```python
from build123d import *

# Parameters (mm, degrees)
SKETCH1_W           = 120
SKETCH1_H           = 110
SKETCH1_W_2         = 98
SKETCH1_H_2         = 40.5
BOSS_EXTRUDE1_DEPTH = 5
SKETCH2_R           = 1.25
CUT_EXTRUDE1_DEPTH  = 4
SKETCH3_R           = 3.5
CUT_EXTRUDE2_DEPTH  = 99.208006293
SKETCH4_R           = 4
CUT_EXTRUDE3_DEPTH  = 99.208006293
SKETCH5_R           = 4.5
CUT_EXTRUDE4_DEPTH  = 2
SKETCH6_W           = 120
SKETCH6_H           = 110
SKETCH6_W_2         = 110
SKETCH6_H_2         = 101
BOSS_EXTRUDE3_DEPTH = 20
SKETCH7_R           = 2.25
CUT_EXTRUDE5_DEPTH  = 143.785021974
BOSS_EXTRUDE5_START = 4
SKETCH9_R           = 1.25
BOSS_EXTRUDE5_DEPTH = 4
BOSS_EXTRUDE6_START = 11
SKETCH10_R          = 1.25
BOSS_EXTRUDE6_DEPTH = 11
BOSS_EXTRUDE7_DEPTH = 4


with BuildPart() as part:
    # Sketch1 → Boss-Extrude1 (new body)
    with BuildSketch(Plane(origin=(0, 0, 0), x_dir=(1, 0, 0), z_dir=(0, 1, 0))):
        with Locations((3.5, -19.75)):
            Rectangle(SKETCH1_W, SKETCH1_H)
        Rectangle(SKETCH1_W_2, SKETCH1_H_2, mode=Mode.SUBTRACT)
    extrude(amount=BOSS_EXTRUDE1_DEPTH)

    # Sketch2 → Cut-Extrude1 (cut)
    with BuildSketch(Plane.XZ):
        with Locations(Location((-46.5, 27.5, 0), (0, 0, 270))):
            Circle(SKETCH2_R)
        with Locations(Location((46.5, 27.5, 0), (0, 0, 270))):
            Circle(SKETCH2_R)
        with Locations(Location((46.5, -27.5, 0), (0, 0, 270))):
            Circle(SKETCH2_R)
        with Locations(Location((-46.5, -27.5, 0), (0, 0, 270))):
            Circle(SKETCH2_R)
        with Locations(Location((-46.5, 33.5, 0), (0, 0, 270))):
            Circle(SKETCH2_R)
        with Locations(Location((50.5, 33.5, 0), (0, 0, 270))):
            Circle(SKETCH2_R)
        with Locations(Location((50.5, 66.5, 0), (0, 0, 270))):
            Circle(SKETCH2_R)
        with Locations(Location((-46.5, 66.5, 0), (0, 0, 270))):
            Circle(SKETCH2_R)
    extrude(amount=-CUT_EXTRUDE1_DEPTH, mode=Mode.SUBTRACT)

    # Sketch3 → Cut-Extrude2 (cut, through all)
    with BuildSketch(Plane(origin=(0, 5, 0), x_dir=(1, 0, 0), z_dir=(0, 1, 0))):
        with Locations(Location((43, -35, 0), (0, 0, 270))):
            Circle(SKETCH3_R)
        with Locations(Location((43, -49, 0), (0, 0, 270))):
            Circle(SKETCH3_R)
        with Locations(Location((43, -63, 0), (0, 0, 270))):
            Circle(SKETCH3_R)
        with Locations(Location((26.5, -49, 0), (0, 0, 270))):
            Circle(SKETCH3_R)
        with Locations(Location((10, -49, 0), (0, 0, 270))):
            Circle(SKETCH3_R)
        with Locations(Location((10, -35, 0), (0, 0, 270))):
            Circle(SKETCH3_R)
        with Locations(Location((10, -63, 0), (0, 0, 270))):
            Circle(SKETCH3_R)
        with Locations(Location((-6.5, -49, 0), (0, 0, 270))):
            Circle(SKETCH3_R)
    extrude(amount=-CUT_EXTRUDE2_DEPTH, mode=Mode.SUBTRACT)

    # Sketch4 → Cut-Extrude3 (cut, through all)
    with BuildSketch(Plane(origin=(0, 5, 0), x_dir=(1, 0, 0), z_dir=(0, 1, 0))):
        with Locations(Location((-39.5, -56, 0), (0, 0, 270))):
            Circle(SKETCH4_R)
    extrude(amount=-CUT_EXTRUDE3_DEPTH, mode=Mode.SUBTRACT)

    # Sketch5 → Cut-Extrude4 (cut)
    with BuildSketch(Plane.XZ):
        with Locations(Location((43, 63, 0), (0, 0, 270))):
            Circle(SKETCH5_R)
        with Locations(Location((43, 49, 0), (0, 0, 270))):
            Circle(SKETCH5_R)
        with Locations(Location((43, 35, 0), (0, 0, 270))):
            Circle(SKETCH5_R)
        with Locations(Location((26.5, 49, 0), (0, 0, 270))):
            Circle(SKETCH5_R)
        with Locations(Location((10, 49, 0), (0, 0, 270))):
            Circle(SKETCH5_R)
        with Locations(Location((10, 35, 0), (0, 0, 270))):
            Circle(SKETCH5_R)
        with Locations(Location((-6.5, 49, 0), (0, 0, 270))):
            Circle(SKETCH5_R)
        with Locations(Location((10, 63, 0), (0, 0, 270))):
            Circle(SKETCH5_R)
    extrude(amount=-CUT_EXTRUDE4_DEPTH, mode=Mode.SUBTRACT)

    # Sketch6 → Boss-Extrude3 (add)
    with BuildSketch(Plane.XZ):
        with Locations((3.5, 19.75)):
            Rectangle(SKETCH6_W, SKETCH6_H)
        with Locations((3.5, 20.25)):
            Rectangle(SKETCH6_W_2, SKETCH6_H_2, mode=Mode.SUBTRACT)
    extrude(amount=BOSS_EXTRUDE3_DEPTH)

    # Sketch7 → Cut-Extrude5 (cut, through all)
    with BuildSketch(Plane(origin=(63.5, 0, 0), x_dir=(0, 0, -1), z_dir=(1, 0, 0))):
        with Locations((22.75, -11)):
            Circle(SKETCH7_R)
    extrude(amount=-CUT_EXTRUDE5_DEPTH, mode=Mode.SUBTRACT)

    # Sketch9 → Boss-Extrude5 (add)
    # profile 1 of 4: a face of its own
    with BuildSketch(Plane.XZ.offset(BOSS_EXTRUDE5_START)):
        with BuildLine():
            Line((-51.5, 30.625), (-46.5, 30.625))
            ThreePointArc((-46.5, 30.625), (-43.375, 27.5), (-46.5, 24.375))
            Line((-46.5, 24.375), (-51.5, 24.375))
            Line((-51.5, 24.375), (-51.5, 30.625))
        make_face()
        with Locations(Location((-46.5, 27.5, 0), (0, 0, 270))):
            Circle(SKETCH9_R, mode=Mode.SUBTRACT)
    # profile 2 of 4: a face of its own
    with BuildSketch(Plane.XZ.offset(BOSS_EXTRUDE5_START)):
        with BuildLine():
            Line((46.5, 30.625), (58.5, 30.625))
            ThreePointArc((58.5, 30.625), (61.625, 27.5), (58.5, 24.375))
            Line((58.5, 24.375), (46.5, 24.375))
            ThreePointArc((46.5, 24.375), (43.375, 27.5), (46.5, 30.625))
        make_face()
        with Locations(Location((46.5, 27.5, 0), (0, 0, 270))):
            Circle(SKETCH9_R, mode=Mode.SUBTRACT)
    # profile 3 of 4: a face of its own
    with BuildSketch(Plane.XZ.offset(BOSS_EXTRUDE5_START)):
        with BuildLine():
            Line((-51.5, -24.375), (-46.5, -24.375))
            ThreePointArc((-46.5, -24.375), (-44.290291309, -25.290291309), (-43.375, -27.5))
            Line((-43.375, -27.5), (-43.375, -30.25))
            Line((-43.375, -30.25), (-51.5, -30.25))
            Line((-51.5, -30.25), (-51.5, -24.375))
        make_face()
        with Locations(Location((-46.5, -27.5, 0), (0, 0, 270))):
            Circle(SKETCH9_R, mode=Mode.SUBTRACT)
    # profile 4 of 4: a face of its own
    with BuildSketch(Plane.XZ.offset(BOSS_EXTRUDE5_START)):
        with BuildLine():
            Line((43.375, -30.25), (43.375, -27.5))
            ThreePointArc((43.375, -27.5), (44.290291309, -25.290291309), (46.5, -24.375))
            Line((46.5, -24.375), (58.5, -24.375))
            Line((58.5, -24.375), (58.5, -30.25))
            Line((58.5, -30.25), (43.375, -30.25))
        make_face()
        with Locations(Location((46.5, -27.5, 0), (0, 0, 270))):
            Circle(SKETCH9_R, mode=Mode.SUBTRACT)
    extrude(amount=-BOSS_EXTRUDE5_DEPTH)

    # Sketch10 → Boss-Extrude6 (add)
    # profile 1 of 4: a face of its own
    with BuildSketch(Plane.XZ.offset(BOSS_EXTRUDE6_START)):
        with BuildLine():
            Line((-46.5, 30.625), (-51.5, 30.625))
            ThreePointArc((-51.5, 30.625), (-54.375, 33.5), (-51.5, 36.375))
            Line((-51.5, 36.375), (-46.5, 36.375))
            ThreePointArc((-46.5, 36.375), (-43.625, 33.5), (-46.5, 30.625))
        make_face()
        with Locations(Location((-46.5, 33.5, 0), (0, 0, 270))):
            Circle(SKETCH10_R, mode=Mode.SUBTRACT)
    # profile 2 of 4: a face of its own
    with BuildSketch(Plane.XZ.offset(BOSS_EXTRUDE6_START)):
        with BuildLine():
            Line((50.5, 36.375), (58.5, 36.375))
            ThreePointArc((58.5, 36.375), (61.375, 33.5), (58.5, 30.625))
            Line((58.5, 30.625), (50.5, 30.625))
            ThreePointArc((50.5, 30.625), (47.625, 33.5), (50.5, 36.375))
        make_face()
        with Locations(Location((50.5, 33.5, 0), (0, 0, 270))):
            Circle(SKETCH10_R, mode=Mode.SUBTRACT)
    # profile 3 of 4: a face of its own
    with BuildSketch(Plane.XZ.offset(BOSS_EXTRUDE6_START)):
        with BuildLine():
            Line((-51.5, 63.625), (-46.5, 63.625))
            ThreePointArc((-46.5, 63.625), (-44.467068004, 64.467068004), (-43.625, 66.5))
            Line((-43.625, 66.5), (-43.625, 70.75))
            Line((-43.625, 70.75), (-51.5, 70.75))
            Line((-51.5, 70.75), (-51.5, 63.625))
        make_face()
        with Locations(Location((-46.5, 66.5, 0), (0, 0, 270))):
            Circle(SKETCH10_R, mode=Mode.SUBTRACT)
    # profile 4 of 4: a face of its own
    with BuildSketch(Plane.XZ.offset(BOSS_EXTRUDE6_START)):
        with BuildLine():
            Line((47.625, 70.75), (47.625, 66.5))
            ThreePointArc((47.625, 66.5), (48.467068004, 64.467068004), (50.5, 63.625))
            Line((50.5, 63.625), (58.5, 63.625))
            Line((58.5, 63.625), (58.5, 70.75))
            Line((58.5, 70.75), (47.625, 70.75))
        make_face()
        with Locations(Location((50.5, 66.5, 0), (0, 0, 270))):
            Circle(SKETCH10_R, mode=Mode.SUBTRACT)
    extrude(amount=-BOSS_EXTRUDE6_DEPTH)

    # Sketch11 → Boss-Extrude7 (add)
    with BuildSketch(Plane.XZ):
        Polygon((-43.625, 33.5), (-43.375, 27.5), (-46.5, 30.625), align=None)
        with BuildLine():
            Line((47.625, 33.5), (50.5, 30.625))
            Line((50.5, 30.625), (45.463150289, 30.447976879))
            ThreePointArc((45.463150289, 30.447976879), (47.029785086, 31.629943897), (47.625, 33.5))
        make_face()
    extrude(amount=BOSS_EXTRUDE7_DEPTH)


solid = part.part
```
The model under review builds one solid part; all positions refer to its coordinate system, in mm. A direction names the side the tool comes from. Round coordinates to 2 decimals unless told otherwise and drop trailing zeros. Order: outer loops, then holes, each group sorted by start corner. A loop starts at its lowest first (then second) coordinate and runs counter-clockwise, first axis right, second up. Notation, with made-up numbers: (41, 0) -> (90, 0) arc R23 cw to (90, 22) -> close; hole circle Ø2 at (-22, 82). An arc over 180 degrees is marked (long way). Use a Markdown table: item, result.
Q1. We need section A-A on z = -22.75. Write out the cut boundary in (x, y), then the cut area to 3 significant figures.
Values:
| item | result |
|---|---|
| outline | (-56.5, -20) -> (-51.5, -20) -> (-51.5, -13.25) -> (-56.5, -13.25) -> close; (-56.5, -8.75) -> (-51.5, -8.75) -> (-51.5, 0) -> (58.5, 0) -> (58.5, -8.75) -> (63.5, -8.75) -> (63.5, 5) -> (-56.5, 5) -> close; (58.5, -20) -> (63.5, -20) -> (63.5, -13.25) -> (58.5, -13.25) -> close |
| area | 755 mm^2 |
Q2. We need section D-D on x = 10. State how many separate pieces and enclosed holes the cut face has, then the cut area to 4 significant figures.
Values:
| item | result |
|---|---|
| separate pieces | 5 |
| enclosed holes | 0 |
| area | 410.5 mm^2 |
Q3. Clearance check with flat-ended pins moving along their axes: P1, Ø10, axis at x = 10.5, z = 49, coming from the -Y side; P2, Ø4.5, axis at x = 11, z = 61.5, coming from the -Y side; P3, Ø2, axis at x = -46.5, z = 33.5, coming from the -Y side. State where each tip first meets the part, or that it passes through.
Values:
| item | result |
|---|---|
| P1 | stops at y = 0 |
| P2 | stops at y = 2 |
| P3 | stops at y = 4 |
Q4. Tool access review of faces 1 (the cylindrical face through (28.865, 3.521, 46.42)), 2 (the flat face through (-43.625, -6, 69)): name each direction out of +Z, -Z, +X, -X, +Y, -Y from which nothing blocks a thin tool from reaching the whole face with its end or side.
Values:
| item | result |
|---|---|
| face 1 | +Y, -Y |
| face 2 | -Y |
Q5. We need section B-B on x = -6.5. Write out the cut boundary in (y, z), then the cut area to 4 significant figures.
Values:
| item | result |
|---|---|
| outline | (-20, -35.25) -> (5, -35.25) -> (5, -20.25) -> (0, -20.25) -> (0, -30.25) -> (-20, -30.25) -> close; (-20, 70.75) -> (0, 70.75) -> (0, 53.5) -> (2, 53.5) -> (2, 52.5) -> (5, 52.5) -> (5, 74.75) -> (-20, 74.75) -> close; (0, 20.25) -> (5, 20.25) -> (5, 45.5) -> (2, 45.5) -> (2, 44.5) -> (0, 44.5) -> close |
| area | 488.5 mm^2 |
Q6. We need section C-C on z = 56. Write out the cut boundary in (x, y).
Values:
| item | result |
|---|---|
| outline | (-56.5, -20) -> (-51.5, -20) -> (-51.5, 0) -> (-43.5, 0) -> (-43.5, 5) -> (-56.5, 5) -> close; (-35.5, 0) -> (58.5, 0) -> (58.5, -20) -> (63.5, -20) -> (63.5, 5) -> (-35.5, 5) -> close |
Q7. Mouldability with a two-part tool opening along X and no side actions: class faces 3 (the flat face through (3, 5, 31)), 4 (the flat face through (6, 2, 49)) as +X half, -X half, draft (parallel to the pull), parting line (faces both ways), or undercut.
Values:
| item | result |
|---|---|
| face 3 | draft |
| face 4 | undercut |
Q8. For line 1 (X direction, y = 3.95, z = 49); line 2 (X direction, y = 1.1, z = 49); line 3 (X direction, y = -6.5, z = 66.5) (3 decimals), list the stretches that pass through material, from the lowest coordinate up.
Values:
| item | result |
|---|---|
| line 1 | x = -56.5 to -10, -3 to 6.5, 13.5 to 23, 30 to 39.5, 46.5 to 63.5 |
| line 2 | x = -56.5 to -11, -2 to 5.5, 14.5 to 22, 31 to 38.5, 47.5 to 63.5 |
| line 3 | x = -56.5 to -47.75, -45.25 to -43.625, 47.625 to 49.25, 51.75 to 63.5 |
